Autodesk Inventor part; units mm, degrees
ref_plane "YZ Plane" through (0, 0, 0) normal (1, 0, 0) x (0, 1, 0)
ref_plane "XZ Plane" through (0, 0, 0) normal (0, 1, 0) x (-1, 0, 0)
ref_plane "XY Plane" through (0, 0, 0) normal (0, 0, 1) x (1, 0, 0)
sketch "Sketch1" plane through (0, 0, 0) normal (1, 0, 0) x (0, 1, 0)
  line L0 (0, 0) -> (88.9, 0)
  line L1 (88.9, 0) -> (88.9, -241.8264)
  line L2 (88.9, -241.8264) -> (0, -241.8264)
  line L3 (0, -241.8264) -> (0, 0)
  line L4 (88.9, 0) -> (0, -51.3264)
  line L5 (88.9, 0) -> (191.5529, 0) construction
  dimension "d0" = 88.9
  dimension "d2" = 150
  dimension "d5" = 190.5
extrude "Extrusion1" add sketch "Sketch1" along normal blind 1.8542 contours L1 L2 L3 L4
sketch "Sketch2" plane through (1.8542, 0, 0) normal (1, 0, 0) x (0, 0, -1)
  line L0 (241.8264, 0) -> (241.8264, 88.9)
  line L1 (51.3264, 0) -> (241.8264, 0)
  line L2 (0, 88.9) -> (51.3264, 0)
  point P0 (0, 0)
  point P1 (82.2382, 16.002)
  point P2 (98.2382, 16.002)
  point P3 (187.2164, 16.002)
  point P4 (203.2164, 16.002)
  point P5 (53.6378, 28.0005)
  point P6 (61.7404, 13.9664)
  dimension "d6" = 16
  dimension "d8" = 16
  dimension "d9" = 16.002
  dimension "d10" = 16.002
  dimension "d11" = 16.002
  dimension "d12" = 16.002
  dimension "d13" = 159.5882
  dimension "d14" = 54.61
  dimension "d22" = 16.002
  dimension "d23" = 16.002
  dimension "d24" = 188.1886
  dimension "d25" = 180.086
hole "Hole1" at (1.8542, 16.002, -82.2382) at (1.8542, 16.002, -98.2382) at (1.8542, 16.002, -187.2164) at (1.8542, 16.002, -203.2164) at (1.8542, 28.0005, -53.6378) at (1.8542, 13.9664, -61.7404) direction (-1, 0, 0) diameter 3.81 depth 10.9728 tip angle 118
sketch "Sketch3" plane through (1.8542, 0, 0) normal (1, 0, 0) x (0, 0, -1)
  line L0 (241.8264, 0) -> (241.8264, 88.9)
  line L1 (51.3264, 0) -> (241.8264, 0)
  point P0 (0, 0)
  point P1 (228.5676, 76.2)
  point P2 (228.5676, 38.1)
  dimension "d26" = 13.2588
  dimension "d27" = 13.2588
  dimension "d28" = 76.2
  dimension "d29" = 38.1
hole "Hole2" at (1.8542, 76.2, -228.5676) at (1.8542, 38.1, -228.5676) direction (-1, 0, 0) diameter 3.81 depth 10.9728 tip angle 118
properties part number "PaddleCollection2.1Casing" material "Polycarbonate, Clear"
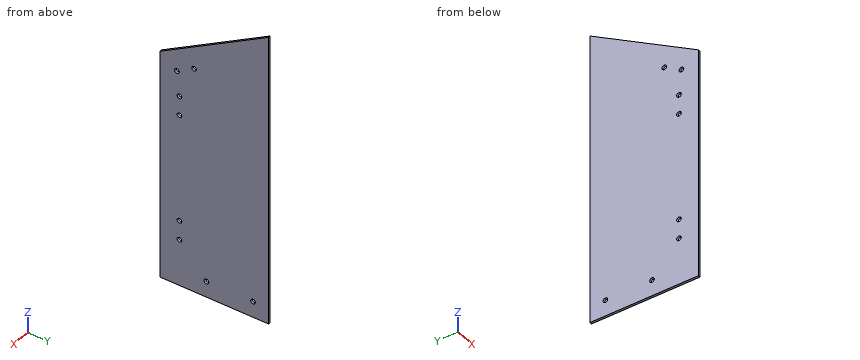
Source: CAD feature listing. Evaluate the final solid. Frame: model axes, mm. Coordinates: 2 decimals unless noted, no trailing zeros. Write each loop counter-clockwise with the first axis right and the second up, starting at its lowest first coordinate (ties: lowest second). Pieces come first, ordered by that corner, then holes. Notation, with made-up numbers: (12.5, 13) - (22.5, 13) arc R26 cw to (22.5, 29) - close; hole circle Ø3 at (79.5, 63.25). An arc over 180 degrees is marked (long way). Answer as a JSON object with one key per item and string values.
Q1. Section query C-C, the plane y = 44.5. Output: boundary loops of the cut face in (x, z).
Ans:
{"outline": "(0, -241.83) - (1.85, -241.83) - (1.85, -25.63) - (0, -25.63) - close"}
Q2. First-contact query: pin 1 Ø3 at (y, z) = (28, -53.64) entering from +X. Flat tip, straight axial feed; report the tip coordinate or a pass-through.
Ans:
{"pin 1": "passes through"}
Q3. Section query A-A, the plane x = 1.55. State how many separate pieces and enclosed holes the cut face has, plus the area to 3 significant figures.
Ans:
{"separate pieces": "1", "enclosed holes": "8", "area": "19,100 mm2"}
Q4. Section query B-B, the plane z = -39.5. Output: boundary loops of the cut face in (x, y), plus the area to 3 significant figures.
Ans:
{"outline": "(0, 20.48) - (1.85, 20.48) - (1.85, 88.9) - (0, 88.9) - close", "area": "127 mm2"}
Q5. Material intervals for line 1 (Y direction, x = 0.1, z = -81); line 2 (Z direction, x = 0.9, y = 27.5); line 3 (Z direction, x = 0.9, y = 79.5), sorted ascending. Write a range as [from, to].
Ans:
{"line 1": "y = [0, 14.55], [17.45, 88.9]", "line 2": "z = [-241.83, -55.48], [-51.8, -35.45]", "line 3": "z = [-241.83, -5.43]"}
